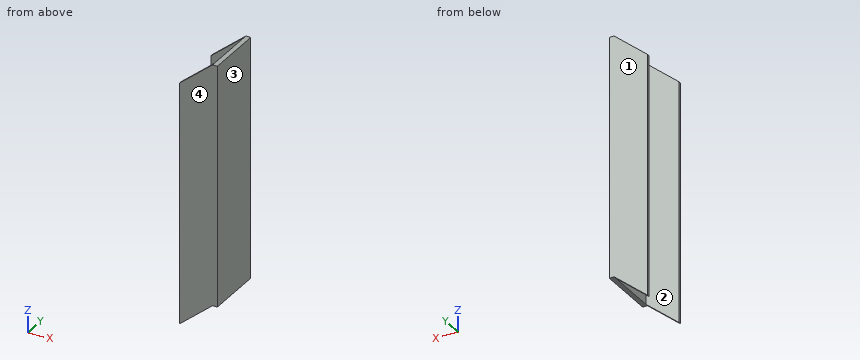
Autodesk Inventor part; units mm, degrees
ref_plane "YZ Plane" through (0, 0, 0) normal (1, 0, 0) x (0, 1, 0)
ref_plane "XZ Plane" through (0, 0, 0) normal (0, 1, 0) x (-1, 0, 0)
ref_plane "XY Plane" through (0, 0, 0) normal (0, 0, 1) x (1, 0, 0)
sketch "Sketch1" plane through (0, 0, 0) normal (1, 0, 0) x (0, 1, 0)
  line L0 (0, 0) -> (-60, 0)
  line L1 (-60, 0) -> (-60, 250)
  line L2 (-60, 250) -> (0, 250)
  line L3 (0, 250) -> (0, 0)
  dimension "d0" = 60
  dimension "d1" = 250
extrude "Extrusion1" add sketch "Sketch1" along normal blind 5
sketch "Sketch2" plane through (5, 0, 0) normal (1, 0, 0) x (0, 0, -1)
  point P0 (0, 0)
sketch "Sketch3" plane through (0, 0, 250) normal (0, 1, 0) x (1, 0, 0)
  line L0 (-34.5249, 250) -> (-35, 250)
  line L1 (0, 250) -> (-34.5249, 278.9698)
  line L2 (0, 250) -> (45.069, 250) construction
  line L3 (-34.5249, 0) -> (-35, 0)
  line L4 (0, 0) -> (-34.5249, 28.9698)
  line L5 (0, 0) -> (45.069, 0) construction
  line L6 (-34.5249, 28.9698) -> (-34.5249, 278.9698)
  line L7 (0, 0) -> (0, 250)
  dimension "d4" = 35
  dimension "d5" = 45.069
  dimension "d6" = 140
  dimension "d7" = 35
  dimension "d8" = 45.069
  dimension "d9" = 140
sketch "Sketch4" plane through (0, 0, 250) normal (0, 1, 0) x (1, 0, 0)
  line L0 (0, 0) -> (0, 250)
extrude "Extrusion2" add sketch "Sketch3" against normal blind 3
sketch "Sketch5" plane through (0, -60, 0) normal (0, -1, 0) x (1, 0, 0)
  line L0 (0, 0) -> (-34.5249, -28.9698)
  line L1 (-34.5249, -28.9698) -> (-34.5249, 221.0302)
  line L2 (-34.5249, 221.0302) -> (0, 250)
  line L3 (0, 250) -> (0, 0)
extrude "Extrusion3" add sketch "Sketch5" against normal blind 3
properties part number "elevation"
Here's how the part is built. I have some questions about the finished solid (model axes, mm). Face numbers are marked on the shaded views. Round coordinates to 2 decimals unless told otherwise and drop trailing zeros. Write each loop counter-clockwise with the first axis right and the second up, starting at its lowest first coordinate (ties: lowest second). Pieces come first, ordered by that corner, then holes.
Q1. If we section it at A-A on z = 70: Write out the boundary of the cut face in (x, y).
Q2. If we mould it in two halves opening along Y, with no side actions, what happens to the marked faces 1, 2, 3 and 4? For each: +Y half, -Y half, draft (parallel to the pull), parting line (faces both ways), or undercut.
Q3. Will these pins go through, and if not, where does the flat tip stop? P1, Ø1.5, axis at y = -29.5, z = 65, coming from the -X side; P2, Ø5.5, axis at x = 3, y = -43, coming from the -Z side.
Q4. Please list where these lines run through material, in increasing order: probe 1 along Y at (x, z) = (-31.5, 30); probe 2 along Z at (x, y) = (3, -51); probe 3 along X at (y, z) = (-15, 177).
Q5. If we section it at C-C on y = -16: Write out the boundary of the cut face in (x, z), plus the area to 3 significant figures.
Q6. If we section it at B-B on x = -23.5: Write out the boundary of the cut face in (y, z).
Answer below:
1. outline: (-34.52, -60) - (5, -60) - (5, 0) - (-34.52, 0) - (-34.52, -3) - (0, -3) - (0, -57) - (-34.52, -57) - close
2. face 1: +Y half
2. face 2: undercut
2. face 3: draft
2. face 4: -Y half
3. P1: stops at x = 0
3. P2: stops at z = 0
4. probe 1: y = -60 to -57, -3 to 0
4. probe 2: z = 0 to 250
4. probe 3: x = 0 to 5
5. outline: (0, 0) - (5, 0) - (5, 250) - (0, 250) - close
5. area: 1,250 mm2
6. outline: (-60, -19.72) - (-57, -19.72) - (-57, 230.28) - (-60, 230.28) - close; (-3, -19.72) - (0, -19.72) - (0, 230.28) - (-3, 230.28) - close
